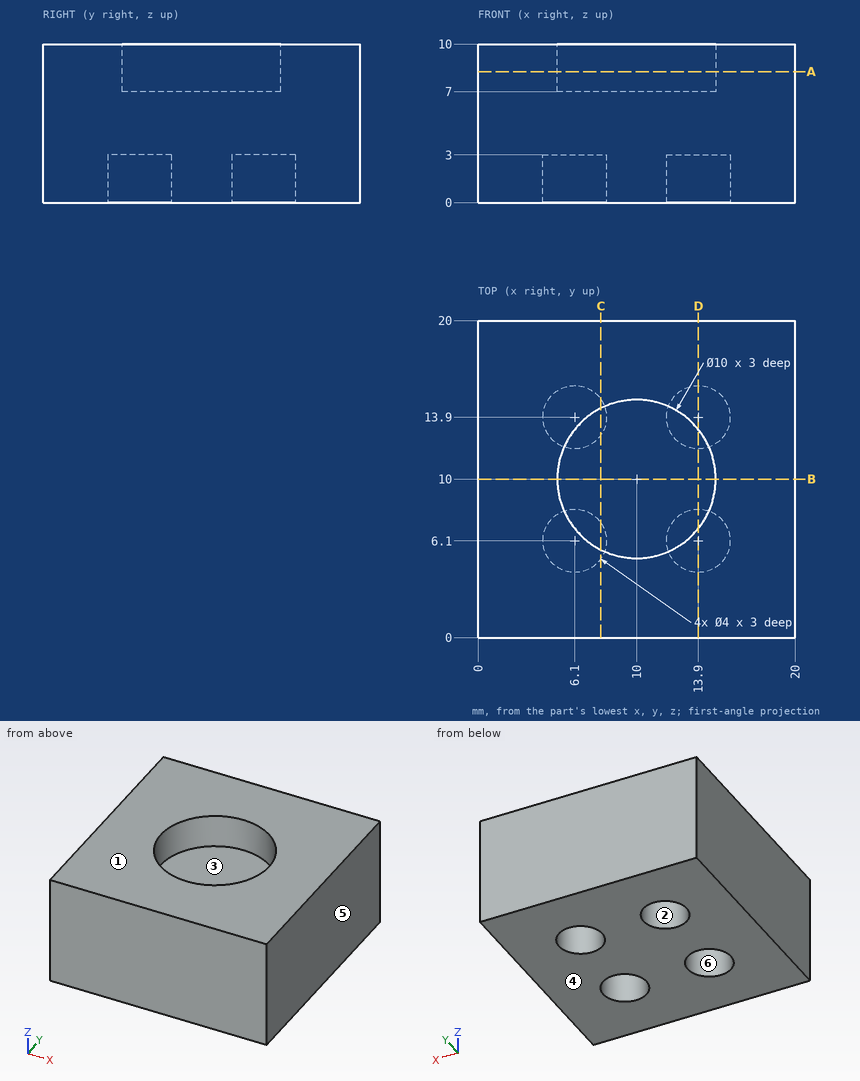
Design review of the part shown in the three views and the two pictorial views. Dimensions are in mm from the part's minimum x, y and z. A direction names the side the tool comes from. Give positions to 0.01 mm unless a question says otherwise; leave off trailing zeros. Write each loop counter-clockwise with the first axis right and the second up, starting at its lowest first coordinate (ties: lowest second). Pieces come first, ordered by that corner, then holes.
Item 1: The part is to be moulded in two halves that separate along X. For the marked faces 4, 5 and 6, say which applies: +X half, -X half, draft (parallel to the pull), parting line (faces both ways), or undercut.
Item 2: Insertion check: P1, Ø1.2, axis at x = 14.5, y = 15, coming from the -Z side. The pin has a flat end and moves straight along its axis. Give the tip position at first contact, or say it passes through.
Item 3: Take a section at A-A (z = 8.25). Give the boundary of the cut face in (x, y), and give its area (3 significant figures).
Item 4: Take a section at B-B (y = 10). Give the boundary of the cut face in (x, z), and give its area (3 significant figures).
Item 5: Take a section at D-D (x = 13.9). Give the boundary of the cut face in (y, z), and give its area (3 significant figures).
Item 6: Take a section at C-C (x = 7.75). Give the boundary of the cut face in (y, z), and give its area (3 significant figures).
Item 7: Wall thickness on probe 1 along Y at (x, z) = (13.9, 2.2); probe 2 along Y at (x, z) = (10, 8.7); probe 3 along X at (y, z) = (5.5, 2.25): over which ranges is each line inside the solid? List them lowest first.
Item 8: Machinability: for the marked faces 1, 2 and 3, which of the approach directions +Z, -Z, +X, -X, +Y, -Y give a long, thin tool a straight path to every point of the face, cutting with its end or side? Answer none if there is none.
Established:
1. face 4: draft
1. face 5: +X half
1. face 6: undercut
2. P1: stops at z = 3
3. outline: (0, 0) - (20, 0) - (20, 20) - (0, 20) - close; hole circle Ø10 at (10, 10)
3. area: 321 mm2
4. outline: (0, 0) - (20, 0) - (20, 10) - (15, 10) - (15, 7) - (5, 7) - (5, 10) - (0, 10) - close
4. area: 170 mm2
5. outline: (0, 0) - (4.1, 0) - (4.1, 3) - (8.1, 3) - (8.1, 0) - (11.9, 0) - (11.9, 3) - (15.9, 3) - (15.9, 0) - (20, 0) - (20, 10) - (13.13, 10) - (13.13, 7) - (6.87, 7) - (6.87, 10) - (0, 10) - close
5. area: 157 mm2
6. outline: (0, 0) - (4.97, 0) - (4.97, 3) - (7.23, 3) - (7.23, 0) - (12.77, 0) - (12.77, 3) - (15.03, 3) - (15.03, 0) - (20, 0) - (20, 10) - (14.47, 10) - (14.47, 7) - (5.53, 7) - (5.53, 10) - (0, 10) - close
6. area: 160 mm2
7. probe 1: y = 0 to 4.1, 8.1 to 11.9, 15.9 to 20
7. probe 2: y = 0 to 5, 15 to 20
7. probe 3: x = 0 to 4.19, 8.01 to 11.99, 15.81 to 20
8. face 1: +Z, +X, -X, +Y, -Y
8. face 2: -Z
8. face 3: +Z
